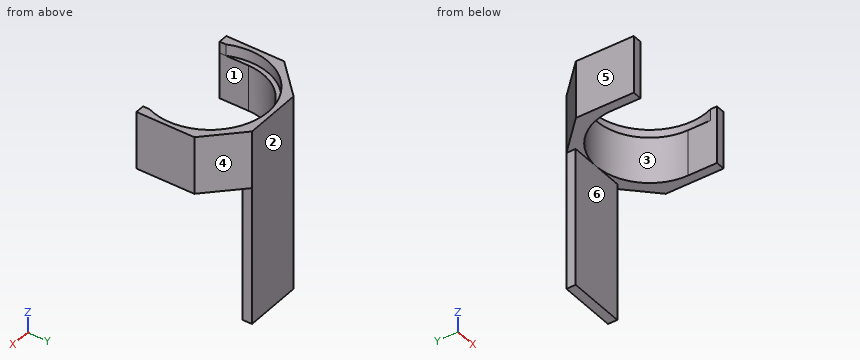
from build123d import *

# Parameters (mm, degrees)
SKETCH_1_W      = 50
SKETCH_1_H      = 8
EXTRUDE_1_DEPTH = 40
EXTRUDE_2_DEPTH = 10


with BuildPart() as part:
    # 扫描1: sweep along a path in 草图2
    with BuildLine(Plane(origin=(0, 0, 0), x_dir=(0, 0, -1), z_dir=(1, 0, 0))) as sweep_1_path:
        Line((0, 55.298323556), (-160, 55.298323556))
    # 草图1 → 扫描1 (sweep)
    with BuildSketch(Plane.XY):
        Rectangle(SKETCH_1_W, SKETCH_1_H)
    sweep(path=sweep_1_path.line)

    # 草图4 → 凸台-拉伸1 (add)
    with BuildSketch(Plane.XY.offset(160)):
        with BuildLine():
            Line((-54, -25), (-25, 4))
            Line((-25, 4), (25, 4))
            Line((25, 4), (54, -25))
            Line((54, -25), (54, -75))
            Line((54, -75), (46, -75))
            Line((46, -75), (46, -50))
            ThreePointArc((46, -50), (0, -4), (-46, -50))
            Line((-46, -50), (-46, -75))
            Line((-46, -75), (-54, -75))
            Line((-54, -75), (-54, -25))
        make_face()
    extrude(amount=-EXTRUDE_1_DEPTH)

    # 草图5 → 凸台-拉伸2 (add)
    with BuildSketch(Plane.XY.offset(160)):
        with BuildLine():
            Line((-46.0046646, -69.584964515), (-46, -75))
            Line((-46, -75), (-54, -75))
            Line((-54, -75), (-54, -25))
            Line((-54, -25), (-25, 4))
            Line((-25, 4), (25, 4))
            Line((25, 4), (54, -25))
            Line((54, -25), (54, -75))
            Line((54, -75), (46, -75))
            Line((46, -75), (46, -69.595917942))
            ThreePointArc((46, -69.595917942), (0.005952648, -3.54e-07), (-46.0046646, -69.584964515))
        make_face()
    extrude(amount=EXTRUDE_2_DEPTH)


solid = part.part
Here's how the part is built. I have some questions about the finished solid (model axes, mm). Face numbers are marked on the shaded views. A direction names the side the tool comes from. Round coordinates to 2 decimals unless told otherwise and drop trailing zeros. Loops run counter-clockwise (first coordinate to the right, second up) from the corner with the lowest first, then second, coordinate; pieces in that order, holes last. Notation, with made-up numbers: (55, 85.25) - (105, 85.25) arc R14 cw to (105, 110.25) - close; hole circle Ø6 at (54, 69). An arc over 180 degrees is marked (long way). One line per question, with ' | ' between items. Start each with the question number.
Q1. We'd pull the mould along X, two halves only. Please class the marked faces 3, 4, 5 and 6: +X half, -X half, draft (parallel to the pull), parting line (faces both ways), or undercut.
Q2. I want a section at B-B (x = 20.5). Write out the boundary of the cut face in (y, z).
Q3. I want a section at A-A (y = -20). Write out the boundary of the cut face in (x, z), then the cut area to 3 significant figures.
Q4. Will these pins go through, and if not, where does the flat tip stop? pin 1 (5 mm diameter, centred on x = -26, z = 65, fed in from -Y); pin 2 (4 mm diameter, centred on y = 0.5, z = 35.5, fed in from -X); pin 3 (4 mm diameter, centred on y = -1.5, z = 69, fed in from +X).
Q5. I want a section at C-C (y = -52). Write out the boundary of the cut face in (x, z), then the cut area to 3 significant figures.
Q6. Please list where these lines run through material, in increasing order: line 1 (X direction, y = -54.5, z = 127.5); line 2 (X direction, y = -50, z = 167); line 3 (Y direction, x = 0, z = 162). Write a range as [from, to].
Q7. For the marked faces 1 and 2, which set-ups out of +Z, -Z, +X, -X, +Y, -Y let a thin tool reach every point of the face, with its end or its side?
Q8. I want a section at D-D (z = 74). Write out the boundary of the cut face in (x, y), then the cut area to 3 significant figures.
Response values:
1) face 3: undercut | face 4: +X half | face 5: -X half | face 6: draft
2) outline: (-8.82, 120) - (-4, 120) - (-4, 0) - (4, 0) - (4, 170) - (-4.4, 170) - (-4.4, 160) - (-8.82, 160) - close
3) outline: (-49, 120) - (-34.87, 120) - (-34.87, 160) - (-40, 160) - (-40, 170) - (-49, 170) - close; (34.87, 120) - (49, 120) - (49, 170) - (40, 170) - (40, 160) - (34.87, 160) - close | area: 1,310 mm²
4) pin 1: stops at y = -4 | pin 2: stops at x = -25 | pin 3: stops at x = 25
5) outline: (-54, 120) - (-46, 120) - (-46, 160) - (-49.96, 160) - (-49.96, 170) - (-54, 170) - close; (46, 120) - (54, 120) - (54, 170) - (49.96, 170) - (49.96, 160) - (46, 160) - close | area: 721 mm²
6) line 1: x = [-54, -46], [46, 54] | line 2: x = [-54, -50], [50, 54] | line 3: y = [0, 4]
7) face 1: +Z, -Z, -Y | face 2: +Z, -Z, +X, -X, +Y
8) outline: (-25, -4) - (25, -4) - (25, 4) - (-25, 4) - close | area: 400 mm²
